Could you check a few things on this model? Use its own coordinates, in mm. Face numbers are marked on the shaded views. A direction names the side the tool comes from. Round coordinates to 2 decimals unless told otherwise and drop trailing zeros. Write each loop counter-clockwise with the first axis right and the second up, starting at its lowest first coordinate (ties: lowest second). Pieces come first, ordered by that corner, then holes. Notation, with made-up numbers: (70, 52) -> (94, 52) arc R18 cw to (94, 72) -> close; hole circle Ø5 at (72, 35.25). An arc over 180 degrees is marked (long way). Answer as CSV lines item,"result". Start each with the question number.
Q1. If I drill on line 1 (Y direction, x = -150, z = 176); line 2 (X direction, y = 37.5, z = -119.5); line 3 (Z direction, x = -35, y = -29.5), over which ranges is the centre line in solid material (lowest first)? Write a range as [from, to].
Q2. For the marked faces 1, 2 and 3, which set-ups out of +Z, -Z, +X, -X, +Y, -Y let a thin tool reach every point of the face, with its end or its side?
Q3. Will these pins go through, and if not, where does the flat tip stop? pin 1 Ø9 at (x, y) = (-205.5, -141.5) entering from -Z; pin 2 Ø19 at (x, z) = (-175, -265.5) entering from +Y; pin 3 Ø5 at (x, z) = (-181.5, -218) entering from +Y.
Q4. Imagine slicing it at B-B on y = 114.5. Please give me the cut outline in (x, z), and give its area (3 significant figures).
Q5. Imagine slicing it at C-C on z = -454.5. Please give me the cut outline in (x, y), and give its area (3 significant figures).
Q6. Imagine slicing it at D-D on z = 2.5. Please give me the cut outline in (x, y), and give its area (3 significant figures).
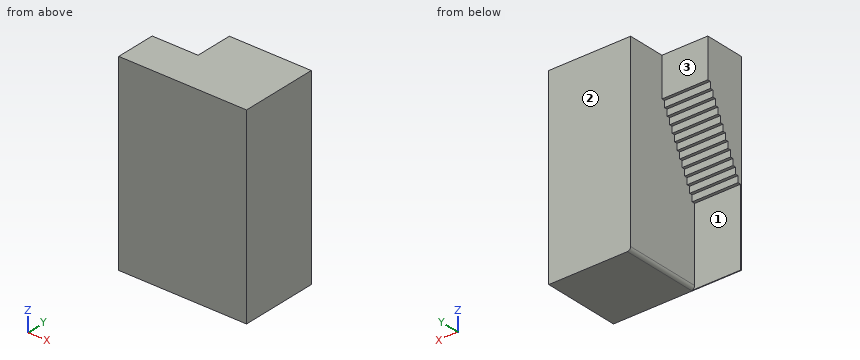
from build123d import *

# Parameters (mm, degrees)
BOSS_EXTRUDE1_DEPTH = 280
SKETCH2_W           = 280
SKETCH2_H           = 5
BOSS_EXTRUDE2_DEPTH = 497.896133892
SKETCH3_W           = 280
SKETCH3_H           = 246.044177264
BOSS_EXTRUDE3_DEPTH = 200
SKETCH4_W           = 280
SKETCH4_H           = 4.725360331
BOSS_EXTRUDE4_DEPTH = 467.31
SKETCH5_W           = 1165.206133892
SKETCH5_H           = 476.142057012
BOSS_EXTRUDE5_DEPTH = 500
FILLET1_R           = 20


with BuildPart() as part:
    # Sketch1 → Boss-Extrude1 (new body)
    with BuildSketch(Plane(origin=(0, 0, 0), x_dir=(0, 0, -1), z_dir=(1, 0, 0))):
        Polygon((-98.3, 73.71314577), (-60, 73.71314577), (-60, 55.21314577), (-21.703866108, 54.668968506), (-21.703866108, 36.168968506), (16.596133892, 36.168968506), (16.596133892, 17.668968506), (54.896133892, 17.668968506), (54.896133892, -0.831031494), (93.196133892, -0.831031494), (93.196133892, -19.331031494), (131.496133892, -19.331031494), (131.496133892, -37.831031494), (169.796133892, -37.831031494), (169.796133892, -56.331031494), (208.096133892, -56.331031494), (208.096133892, -74.831031494), (246.396133892, -74.831031494), (246.396133892, -93.331031494), (284.696133892, -93.331031494), (284.696133892, -111.831031494), (322.996133892, -111.831031494), (322.996133892, -130.331031494), (361.296133892, -130.331031494), (361.296133892, -148.831031494), (399.596133892, -148.831031494), (399.596133892, -167.331031494), (-98.3, -167.331031494), align=None)
    extrude(amount=-BOSS_EXTRUDE1_DEPTH)

    # Sketch2 → Boss-Extrude2 (add)
    with BuildSketch(Plane.XY.offset(98.3)):
        with Locations((-140, -169.831031494)):
            Rectangle(SKETCH2_W, SKETCH2_H)
    extrude(amount=-BOSS_EXTRUDE2_DEPTH)

    # Sketch3 → Boss-Extrude3 (add)
    with BuildSketch(Plane.XY.offset(98.3)):
        with Locations((-140, -49.308942862)):
            Rectangle(SKETCH3_W, SKETCH3_H)
    extrude(amount=BOSS_EXTRUDE3_DEPTH)

    # Sketch4 → Boss-Extrude4 (add)
    with BuildSketch(Plane(origin=(0, 0, -399.596133892), x_dir=(-1, 0, 0), z_dir=(0, 0, -1))):
        with Locations((140, -169.968351329)):
            Rectangle(SKETCH4_W, SKETCH4_H)
    extrude(amount=BOSS_EXTRUDE4_DEPTH)

    # Sketch5 → Boss-Extrude5 (add)
    with BuildSketch(Plane(origin=(0, 0, 0), x_dir=(0, 0, -1), z_dir=(1, 0, 0))):
        with Locations((284.303066946, 65.739997012)):
            Rectangle(SKETCH5_W, SKETCH5_H)
    extrude(amount=BOSS_EXTRUDE5_DEPTH)

    # Fillet1
    fillet1_edges = [part.edges().sort_by_distance(p)[0] for p in [
        (0, 68.102677177, -866.906133892),
    ]]
    fillet(fillet1_edges, radius=FILLET1_R)


solid = part.part
Checks:
1,line 1,"[-172.33, 73.71]"
1,line 2,"[0, 500]"
1,line 3,"[-131.5, 298.3]"
2,face 1,"-Z, -X, +Y"
2,face 2,"+Z, -Z, +X, -X, +Y"
2,face 3,"+Z, -Z, -X, +Y"
3,pin 1,"z = -361.3"
3,pin 2,"y = -93.33"
3,pin 3,"y = -74.83"
4,outline,"(0, -846.91) arc R20 ccw to (20, -866.91) -> (500, -866.91) -> (500, 298.3) -> (0, 298.3) -> close"
4,area,"583,000 mm^2"
5,outline,"(-280, -172.33) -> (500, -172.33) -> (500, 303.81) -> (0, 303.81) -> (0, -167.61) -> (-280, -167.61) -> close"
5,area,"239,000 mm^2"
6,outline,"(-280, -172.33) -> (500, -172.33) -> (500, 303.81) -> (0, 303.81) -> (0, 36.17) -> (-280, 36.17) -> close"
6,area,"296,000 mm^2"
